```python
from build123d import *

# Parameters (mm, degrees)
SKETCH004_R     = 4.1
PAD002_DEPTH    = 10
SKETCH005_R     = 11
POCKET001_DEPTH = 7
PAD_DEPTH       = 7
FILLET_R        = 3
SKETCH002_R     = 4.1
PAD001_DEPTH    = 10
SKETCH003_R     = 11
POCKET_DEPTH    = 7


with BuildPart() as pocket001:
    # Sketch004 → Pad002 (new body)
    with BuildSketch(Plane.XZ.offset(15)):
        with BuildLine():
            Line((-15, 7), (15, 7))
            Line((15, 7), (15, 27))
            ThreePointArc((15, 27), (0, 42.000006), (-15, 27))
            Line((-15, 7), (-15, 27))
        make_face()
        with Locations((0, 27.000006)):
            Circle(SKETCH004_R, mode=Mode.SUBTRACT)
    extrude(amount=PAD002_DEPTH)

    # Sketch005 → Pocket001 (cut)
    with BuildSketch(Plane(origin=(0, -15, 0), x_dir=(1, 0, 0), z_dir=(0, 1, 0))):
        with Locations((0, -27.000006)):
            Circle(SKETCH005_R)
    extrude(amount=-POCKET001_DEPTH, mode=Mode.SUBTRACT)


with BuildPart() as grundplatte001:
    # Sketch → Pad (new body)
    with BuildSketch(Plane.XY):
        Polygon((-36, 15.5), (-36, -15.5), (-26, -25.5), (26, -25.5), (36, -15.5), (36, 15.5), align=None)
        with BuildLine():
            Line((-32.53033, 9.500002), (-32.53033, 5.5))
            ThreePointArc((-32.53033, 5.5), (-31, 3.96967), (-29.46967, 5.5))
            Line((-29.46967, 9.500002), (-29.46967, 5.5))
            ThreePointArc((-29.46967, 9.500002), (-31, 11.03033), (-32.53033, 9.500002))
        make_face(mode=Mode.SUBTRACT)
        with BuildLine():
            Line((-32.55, -10.499998), (-32.55, -14.5))
            ThreePointArc((-32.55, -14.5), (-31, -16.05), (-29.45, -14.5))
            Line((-29.45, -10.499998), (-29.45, -14.5))
            ThreePointArc((-29.45, -10.499998), (-31, -8.95), (-32.55, -10.499998))
        make_face(mode=Mode.SUBTRACT)
        with BuildLine():
            Line((29.45, -10.500011), (29.45, -14.500004))
            ThreePointArc((29.45, -14.500004), (31, -16.05), (32.55, -14.500004))
            Line((32.55, -14.500004), (32.55, -10.500011))
            ThreePointArc((32.55, -10.500011), (31, -8.95), (29.45, -10.500011))
        make_face(mode=Mode.SUBTRACT)
        with BuildLine():
            Line((32.55, 9.500002), (32.55, 5.5))
            ThreePointArc((29.45, 5.5), (31, 3.95), (32.55, 5.5))
            Line((29.45, 9.500002), (29.45, 5.5))
            ThreePointArc((32.55, 9.500002), (31, 11.05), (29.45, 9.500002))
        make_face(mode=Mode.SUBTRACT)
    extrude(amount=PAD_DEPTH)

    # Fillet
    fillet_edges = [grundplatte001.edges().sort_by_distance(p)[0] for p in [
        (26, -25.5, 3.5),
        (-26, -25.5, 3.5),
        (36, -15.5, 3.5),
        (-36, -15.5, 3.5),
        (36, 15.5, 3.5),
        (-36, 15.5, 3.5),
    ]]
    fillet(fillet_edges, radius=FILLET_R)


with BuildPart() as fusion001:
    # Fusion001 base: copy of Grundplatte001
    add(grundplatte001.part)

    # Fusion001: union Pocket001
    add(pocket001.part)


with BuildPart() as lagerbock:
    # Sketch002 → Pad001 (new body)
    with BuildSketch(Plane.XZ.offset(-15)):
        with BuildLine():
            Line((-15, 7), (15, 7))
            Line((15, 7), (15, 27))
            ThreePointArc((15, 27), (0, 42.000006), (-15, 27))
            Line((-15, 7), (-15, 27))
        make_face()
        with Locations((0, 27.000006)):
            Circle(SKETCH002_R, mode=Mode.SUBTRACT)
    extrude(amount=PAD001_DEPTH)

    # Sketch003 → Pocket (cut)
    with BuildSketch(Plane.XZ.offset(-5)):
        with Locations((0, 27.000006)):
            Circle(SKETCH003_R)
    extrude(amount=-POCKET_DEPTH, mode=Mode.SUBTRACT)


with BuildPart() as fusion002:
    # Fusion base: copy of Grundplatte001
    add(grundplatte001.part)

    # Fusion: union Lagerbock
    add(lagerbock.part)

    # Fusion002: union Fusion001
    add(fusion001.part)


solid = fusion002.part
```
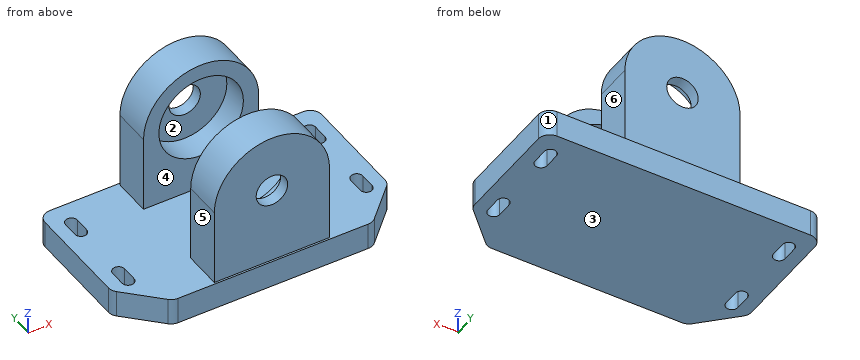
Can you work these out from the model? Positions are in its coordinate system, mm. Face numbers are marked on the shaded views. A direction names the side the tool comes from. Round coordinates to 2 decimals unless told otherwise and drop trailing zeros. Loops run counter-clockwise (first coordinate to the right, second up) from the corner with the lowest first, then second, coordinate; pieces in that order, holes last. Notation, with made-up numbers: (50.25, -25.5) -> (97.25, -25.5) arc R21 cw to (97.25, 5.5) -> close; hole circle Ø4 at (0, -4). An arc over 180 degrees is marked (long way). Answer in a Markdown table with one row per item.
Item 1: Will these pins go through, and if not, where does the flat tip stop? P1, Ø24, axis at x = -4.5, z = 29, coming from the -Y side; P2, Ø1, axis at x = 26, y = -2, coming from the +Z side; P3, Ø5, axis at y = 11, z = 16, coming from the +X side; P4, Ø2, axis at x = -7, y = -20, coming from the -Z side.
Answer block:
| item | result |
|---|---|
| P1 | y = -25 |
| P2 | z = 7 |
| P3 | x = 15 |
| P4 | z = 0 |
Item 2: We'd pull the mould along Y, two halves only. Please class the marked faces 1, 2 and 3: released by +Y, released by -Y, zero draft, split by the parting line, or undercut.
Answer block:
| item | result |
|---|---|
| face 1 | released by +Y |
| face 2 | undercut |
| face 3 | zero draft |
Item 3: On a 3-axis mill with a long thin cutter (end or side, diameter ignored), from which of +Z, -Z, +X, -X, +Y, -Y can I reach the whole of each face in a straight line? I mean the marked faces 4, 5 and 6. Say none if no direction works.
Answer block:
| item | result |
|---|---|
| face 4 | +Z, +X, -X |
| face 5 | +Z, -X, +Y, -Y |
| face 6 | +Z, +X, +Y, -Y |
Item 4: Suppose I cut it at B-B, the plane y = 6.5. List the corners of the cut face in (x, z) for me.
Answer block:
| item | result |
|---|---|
| outline | (-36, 0) -> (-32.53, 0) -> (-32.53, 7) -> (-36, 7) -> close; (-29.47, 0) -> (29.45, 0) -> (29.45, 7) -> (15, 7) -> (15, 27) arc R15 ccw to (-15, 27) -> (-15, 7) -> (-29.47, 7) -> close; (32.55, 0) -> (36, 0) -> (36, 7) -> (32.55, 7) -> close; hole circle Ø22 at (0, 27) |
Item 5: Suppose I cut it at C-C, the plane z = 8. List the corners of the cut face in (x, y) for me.
Answer block:
| item | result |
|---|---|
| outline | (-15, -25) -> (15, -25) -> (15, -15) -> (-15, -15) -> close; (-15, 5) -> (15, 5) -> (15, 15) -> (-15, 15) -> close |
Item 6: Suppose I cut it at A-A, the plane x = -31. List the corners of the cut face in (y, z) for me.
Answer block:
| item | result |
|---|---|
| outline | (-20.5, 0) -> (-16.05, 0) -> (-16.05, 7) -> (-20.5, 7) -> close; (-8.95, 0) -> (3.97, 0) -> (3.97, 7) -> (-8.95, 7) -> close; (11.03, 0) -> (15.5, 0) -> (15.5, 7) -> (11.03, 7) -> close |
Item 7: Suppose I cut it at D-D, the plane x = 31. List the corners of the cut face in (y, z) for me.
Answer block:
| item | result |
|---|---|
| outline | (-20.5, 0) -> (-16.05, 0) -> (-16.05, 7) -> (-20.5, 7) -> close; (-8.95, 0) -> (3.95, 0) -> (3.95, 7) -> (-8.95, 7) -> close; (11.05, 0) -> (15.5, 0) -> (15.5, 7) -> (11.05, 7) -> close |
Item 8: If I drill on probe 1 along Z at (x, y) = (0, 7); probe 2 along Z at (x, y) = (0, -24.2); probe 3 along Y at (x, z) = (-7.5, 19.5), over which ranges is the centre line in solid material (lowest first)?
Answer block:
| item | result |
|---|---|
| probe 1 | 0 to 16, 38 to 42 |
| probe 2 | 0 to 22.9, 31.1 to 42 |
| probe 3 | -25 to -22, 12 to 15 |
